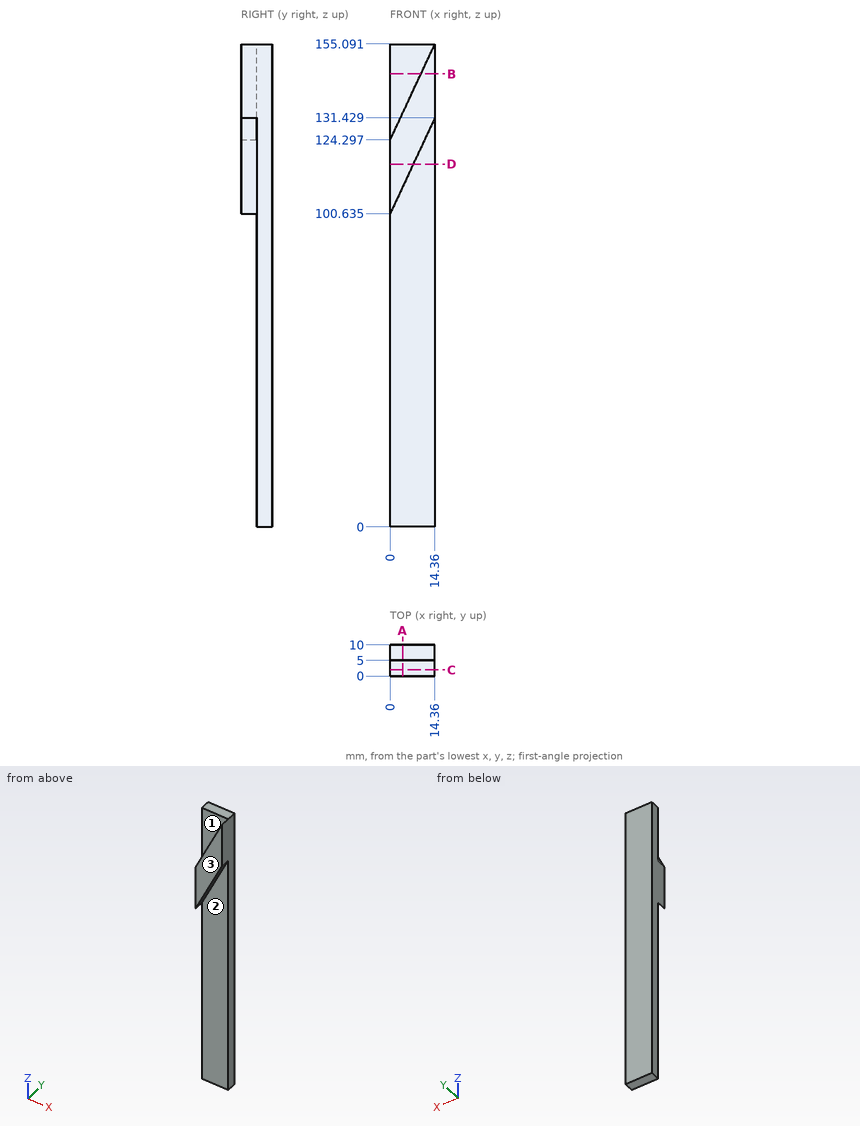
Answer from the drawing. Dimensions are ordinates in mm from the lowest x, y and z of the part. A direction names the side the tool comes from. Give positions to 0.01 mm unless a question says otherwise; leave off trailing zeros. Loops run counter-clockwise (first coordinate to the right, second up) from the corner with the lowest first, then second, coordinate; pieces in that order, holes last. Notation, with made-up numbers: (15.5, -13.5) -> (39.5, -13.5) arc R18 ccw to (39.5, 21.5) -> close; hole circle Ø9 at (83, -16.5). An arc over 180 degrees is marked (long way). Answer as CSV lines item,"result".
Item 1: Find section C-C on y = 2. Give the vertices of the cut face in (x, z) (1 decimal).
Returned:
outline,"(0, 100.6) -> (14.4, 131.4) -> (14.4, 155.1) -> (0, 124.3) -> close"
Item 2: Consider line 1 (Y direction, x = 10.5, z = 8.5); line 2 (Z direction, x = 11.25, y = 2) (1 decimal); line 3 (Z direction, x = 9.75, y = 2.5) (1 decimal). Determine where each line is inside the solid, lowest interval first. Write a range as [from, to].
Returned:
line 1,"y = [5, 10]"
line 2,"z = [124.8, 148.4]"
line 3,"z = [121.5, 145.2]"
Item 3: Find section B-B on z = 145.5. Give the vertices of the cut face in (x, y).
Returned:
outline,"(0, 5) -> (9.89, 5) -> (9.89, 0) -> (14.36, 0) -> (14.36, 10) -> (0, 10) -> close"
Item 4: This flat-tipped pin is pushed along its axis until it touches: pin 1 (4.5 mm diameter, centred on x = 7.5, z = 84, fed in from -Y). Where does it stop, or does it pass through?
Returned:
pin 1,"stops at y = 5"
Item 5: For the marked faces 1, 2 and 3, determine the directions among +Z, -Z, +X, -X, +Y, -Y from which every point of the face is accessible in a straight line to the end or side of a thin tool.
Returned:
face 1,"+Z, -X, -Y"
face 2,"-Z, +X, -Y"
face 3,"+Z, -Z, +X, -X, -Y"
Item 6: Find section A-A on x = 4. Give the vertices of the cut face in (y, z) (1 decimal).
Returned:
outline,"(0, 109.2) -> (5, 109.2) -> (5, 0) -> (10, 0) -> (10, 155.1) -> (5, 155.1) -> (5, 132.9) -> (0, 132.9) -> close"
Item 7: Find section D-D on z = 116.5. Give the vertices of the cut face in (x, y), plus the area to 3 significant figures.
Returned:
outline,"(0, 0) -> (7.4, 0) -> (7.4, 5) -> (14.36, 5) -> (14.36, 10) -> (0, 10) -> close"
area,"109 mm²"
